Check sheet for the drawn part. Datum: minimum x, y, z corner. Units: mm. Round coordinates to 2 decimals unless told otherwise and drop trailing zeros. Write each loop counter-clockwise with the first axis right and the second up, starting at its lowest first coordinate (ties: lowest second). Pieces come first, ordered by that corner, then holes. Notation, with made-up numbers: (51, 79) -> (73, 79) arc R15 ccw to (73, 104) -> close; hole circle Ø8 at (-0.5, -9). An arc over 180 degrees is marked (long way). One line per item, written item: value. Start each with the question number.
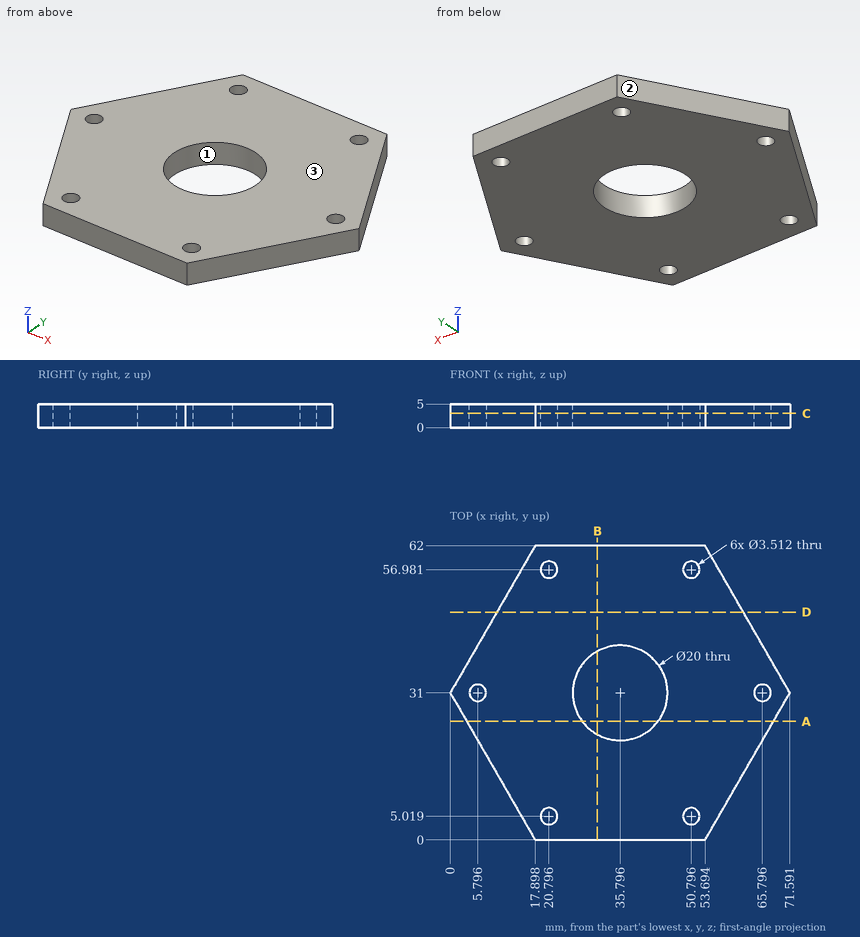
1. Cross-section at C-C (z = 3.05). Record the cut outline in (x, y) (1 decimal).
2. Cross-section at D-D (y = 48). Record the cut outline in (x, z) (1 decimal).
3. Material ranges on probe 1 along Y at (x, z) = (21, 4.8) (1 decimal); probe 2 along X at (y, z) = (56, 4.5) (1 decimal); probe 3 along X at (y, z) = (5.5, 4.5) (1 decimal), recorded low to high.
4. Cross-section at B-B (x = 31). Record the cut outline in (y, z) (1 decimal), plus the area to 3 significant figures.
5. Release check for a two-part mould opening along Y. For the marked faces 1, 2 and 3 record: +Y half, -Y half, draft (parallel to the pull), parting line (faces both ways), or undercut.
6. Cross-section at A-A (y = 25). Record the cut outline in (x, z) (1 decimal).
7. Depth check by flat-ended pin: pin 1 Ø3 at (x, y) = (65.8, 31) entering from +Z; pin 2 Ø3 at (y, z) = (16.5, 1) entering from -X (1 decimal); pin 3 Ø1.5 at (y, z) = (35.5, 4) entering from -X (1 decimal). Enter the tip coordinate at first touch or a pass-through.
Working result:
1. outline: (0, 31) -> (17.9, 0) -> (53.7, 0) -> (71.6, 31) -> (53.7, 62) -> (17.9, 62) -> close; hole circle Ø3.5 at (5.8, 31); hole circle Ø3.5 at (20.8, 5); hole circle Ø3.5 at (20.8, 57); hole circle Ø20 at (35.8, 31); hole circle Ø3.5 at (50.8, 5); hole circle Ø3.5 at (50.8, 57); hole circle Ø3.5 at (65.8, 31)
2. outline: (9.8, 0) -> (61.8, 0) -> (61.8, 5) -> (9.8, 5) -> close
3. probe 1: y = 0 to 3.3, 6.8 to 55.2, 58.7 to 62
3. probe 2: x = 14.4 to 19.3, 22.3 to 49.3, 52.3 to 57.2
3. probe 3: x = 14.7 to 19.1, 22.5 to 49.1, 52.5 to 56.9
4. outline: (0, 0) -> (22.2, 0) -> (22.2, 5) -> (0, 5) -> close; (39.8, 0) -> (62, 0) -> (62, 5) -> (39.8, 5) -> close
4. area: 222 mm^2
5. face 1: undercut
5. face 2: +Y half
5. face 3: draft
6. outline: (3.5, 0) -> (27.8, 0) -> (27.8, 5) -> (3.5, 5) -> close; (43.8, 0) -> (68.1, 0) -> (68.1, 5) -> (43.8, 5) -> close
7. pin 1: passes through
7. pin 2: stops at x = 7.5
7. pin 3: stops at x = 2.2
